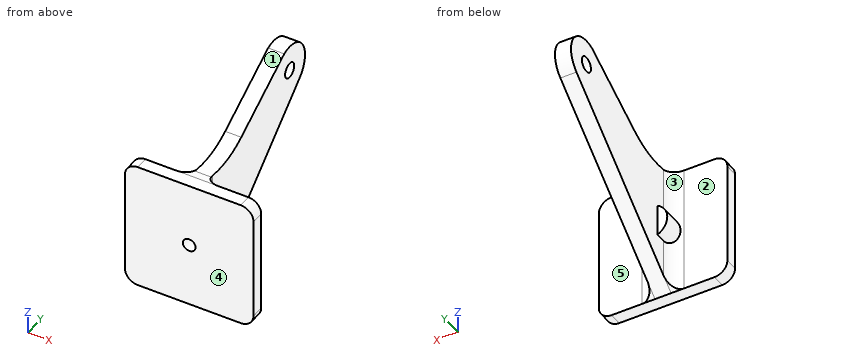
```python
from build123d import *

# Parameters (mm, degrees)
SKETCH1_W           = 25.4
SKETCH1_H           = 25.4
BOSS_EXTRUDE1_DEPTH = 2.54
SKETCH3_R           = 1.5
BOSS_EXTRUDE2_DEPTH = 1.5875
FILLET1_START       = -12.7000001
FILLET1_DEPTH       = 25.4000001
FILLET1_START_2     = -5
FILLET1_2_DEPTH     = 10
FILLET2_R           = 2.54
SKETCH4_R           = 3.5
BOSS_EXTRUDE3_DEPTH = 7
SKETCH5_R           = 1.25
CUT_EXTRUDE1_DEPTH  = 6.35


with BuildPart() as part:
    # Sketch1 → Boss-Extrude1 (new body)
    with BuildSketch(Plane(origin=(0, 0, 0), x_dir=(1, 0, 0), z_dir=(0, 1, 0))):
        Rectangle(SKETCH1_W, SKETCH1_H)
    extrude(amount=BOSS_EXTRUDE1_DEPTH)

    # Sketch3 → Boss-Extrude2 (add, symmetric)
    with BuildSketch(Plane(origin=(0, 0, 0), x_dir=(0, 0, -1), z_dir=(1, 0, 0))):
        with BuildLine():
            Line((-22.53488, 28.69184), (-14.109077454, 14.518123111))
            ThreePointArc((-14.109077454, 14.518123111), (-12.301446379, 9.646212675), (-12.336895325, 4.449888515))
            Line((-12.336895325, 4.449888515), (-12.7, 2.54))
            Line((-12.7, 2.54), (12.7, 2.54))
            Line((12.7, 2.54), (-13.91324895, 33.774637509))
            ThreePointArc((-13.91324895, 33.774637509), (-20.359903271, 34.856128324), (-22.53488, 28.69184))
        make_face()
        with Locations((-17.78, 30.48)):
            Circle(SKETCH3_R, mode=Mode.SUBTRACT)
    extrude(amount=BOSS_EXTRUDE2_DEPTH, both=True)

    # Fillet1: read off the stored shape, not the designer's step
    # Fillet1 outline → Fillet1 (add)
    with BuildSketch(Plane.XY.offset(FILLET1_START)):
        with BuildLine():
            ThreePointArc((-1.5875, 5.08), (-2.331448776, 3.283948776), (-4.1275, 2.54))
            Line((-4.1275, 2.54), (-1.5875, 2.54))
            Line((-1.5875, 2.54), (-1.5875, 5.08))
        make_face()
        with BuildLine():
            Line((1.5875, 2.54), (4.1275, 2.54))
            ThreePointArc((4.1275, 2.54), (2.331448776, 3.283948776), (1.5875, 5.08))
            Line((1.5875, 5.08), (1.5875, 2.54))
        make_face()
    extrude(amount=FILLET1_DEPTH)

    # Fillet1 2 outline → Fillet1 2 (cut)
    with BuildSketch(Plane.YZ.offset(FILLET1_START_2)):
        Polygon((5.08, -10.535811211), (2.54, -12.7), (5.08, -12.7000001), align=None)
        with BuildLine():
            Line((5.08, 12.7), (2.54, 12.7))
            Line((2.54, 12.7), (4.449888515, 12.336895325))
            ThreePointArc((4.449888515, 12.336895325), (4.764360857, 12.280707955), (5.08, 12.231496116))
            Line((5.08, 12.231496116), (5.08, 12.7))
        make_face()
    extrude(amount=FILLET1_2_DEPTH, mode=Mode.SUBTRACT)

    # Fillet2
    fillet2_edges = [part.edges().sort_by_distance(p)[0] for p in [
        (12.7, 1.27, -12.7),
        (12.7, 1.27, 12.7),
        (-12.7, 1.27, 12.7),
        (-12.7, 1.27, -12.7),
    ]]
    fillet(fillet2_edges, radius=FILLET2_R)

    # Sketch4 → Boss-Extrude3 (add)
    with BuildSketch(Plane.XZ):
        Circle(SKETCH4_R)
    extrude(amount=-BOSS_EXTRUDE3_DEPTH)

    # Sketch5 → Cut-Extrude1 (cut)
    with BuildSketch(Plane.XZ):
        with Locations(Location((0, 0, 0), (0, 0, 270))):
            Circle(SKETCH5_R)
    extrude(amount=-CUT_EXTRUDE1_DEPTH, mode=Mode.SUBTRACT)


solid = part.part
```
Geometry: final body of the model. Coordinates: model frame, mm. Face numbers are marked on the shaded views. A direction names the side the tool comes from. Coordinates: 2 decimals unless noted, no trailing zeros. Write each loop counter-clockwise with the first axis right and the second up, starting at its lowest first coordinate (ties: lowest second). Pieces come first, ordered by that corner, then holes. Notation, with made-up numbers: M 0,55.5 L 41,55.5 A19 cw 41,74.5 Z; hole C 15.5,52.25 d6. An arc over 180 degrees is marked long. Use CSV: the item, a comma, the result in double quotes. Start each with the question number.
1. Cut plane B-B on z = 17.78. Return the cut outline in (x, y), plus the area to 3 significant figures.
2. Ray query, probe 1 along X at (y, z) = (2.75, 0); probe 2 along X at (y, z) = (12, 1.5); probe 3 along Y at (x, z) = (-5, -4.5). Return the intervals inside material, ascending.
3. Cut plane D-D on x = 9. Return the cut outline in (y, z).
4. Cut plane A-A on y = 30.48. Return the cut outline in (x, z), plus the area to 3 significant figures.
5. Cut plane C-C on z = 11. Return the cut outline in (x, y), plus the area to 3 significant figures.
6. Reachability of the marked faces 1, 2, 3, 4 and 5 from +Z, -Z, +X, -X, +Y, -Y: full face, straight path, thin tool, end or side. Return the list, or none.
7. First-contact query: P1, Ø1.5, axis at x = 0, z = 0, coming from the -Y side; P2, Ø7, axis at x = -10, z = 2, coming from the +Y side; P3, Ø3.5, axis at y = 30.48, z = 17.78, coming from the +X side. Flat tips, straight axial feed; report the tip coordinate or a pass-through.
Entries:
1,outline,"M -1.59,20.69 L 1.59,20.69 L 1.59,28.98 L -1.59,28.98 Z; M -1.59,31.98 L 1.59,31.98 L 1.59,35.56 L -1.59,35.56 Z"
1,area,"37.7 mm²"
2,probe 1,"-3.5 to -1.25, 1.25 to 3.5"
2,probe 2,"-1.59 to 1.59"
2,probe 3,"0 to 2.54"
3,outline,"M 0,-12.7 L 2.54,-12.7 L 2.54,12.7 L 0,12.7 Z"
4,outline,"M -1.59,11.11 L 1.59,11.11 L 1.59,16.28 L -1.59,16.28 Z; M -1.59,19.28 L 1.59,19.28 L 1.59,22.86 L -1.59,22.86 Z"
4,area,"27.8 mm²"
5,outline,"M -12.56,0 L 12.56,0 L 12.56,2.54 L 4.13,2.54 A2.54 cw 1.59,5.08 L 1.59,30.36 L -1.59,30.36 L -1.59,5.08 A2.54 cw -4.13,2.54 L -12.56,2.54 Z"
5,area,"155 mm²"
6,face 1,"+Z, +X, -X, -Y"
6,face 2,"+Z, -Z, -X, +Y"
6,face 3,"-X, +Y"
6,face 4,"+Z, -Z, +X, -X, -Y"
6,face 5,"+Z, -Z, +X, +Y"
7,P1,"y = 6.35"
7,P2,"y = 2.54"
7,P3,"x = 1.59"
